from build123d import *

# Parameters (mm, degrees)
F0_W     = 80
F0_H     = 25
F0_R     = 7.5
F1_DEPTH = 5
F2_W     = 80
F2_H     = 25
F2_R     = 7.5
F2_W_2   = 5
F2_H_2   = 5
F3_DEPTH = 5


with BuildPart() as f1:
    # F0 (on Top) → F1 (new body)
    with BuildSketch(Plane.XY):
        with Locations((-49.0031225234, 12.5)):
            Rectangle(F0_W, F0_H)
        with Locations((-21.5031225234, 12.5)):
            Circle(F0_R, mode=Mode.SUBTRACT)
    extrude(amount=F1_DEPTH)

    # F2 (on face) → F3 (join)
    with BuildSketch(Plane(origin=(0, 0, 0), x_dir=(1, 0, 0), z_dir=(0, 0, -1))):
        with Locations((-49.0031225234, -12.5)):
            Rectangle(F2_W, F2_H)
        with Locations((-21.5031225234, -12.5)):
            Circle(F2_R, mode=Mode.SUBTRACT)
        with Locations((-21.5031225234, -12.5)):
            Circle(F2_R)
        with Locations((-21.5031225234, -12.5)):
            Rectangle(F2_W_2, F2_H_2, mode=Mode.SUBTRACT)
    extrude(amount=F3_DEPTH)


solid = f1.part
Geometry check sheet. Reference: the model listing, model coordinates, mm. A direction names the side the tool comes from. Round coordinates to 2 decimals unless told otherwise and drop trailing zeros. Order: outer loops, then holes, each group sorted by start corner. A loop starts at its lowest first (then second) coordinate and runs counter-clockwise, first axis right, second up. Notation, with made-up numbers: M -3.5,-37 L 26.5,-37 A31 cw 26.5,-8 Z; hole C 67.5,-24.5 d9. An arc over 180 degrees is marked long. Write each question's results on one line, items separated by ' | '. Start each with the question number.
1. Cross-section at A-A on y = 12.5. Record the boundary of the cut face in (x, z).
2. Cross-section at C-C on y = 16.5. Record the boundary of the cut face in (x, z), plus the area to 3 significant figures.
3. Draft check along X on faces 1 (the face through (-22, 15, -2)), 2 (the face through (-50, 12, -5)), 3 (the face through (-89.003, 13, 0)). Enter one of: pulls with the +X half, pulls with the -X half, needs draft (parallel to the pull), parting line crosses it, or undercut.
4. Cross-section at B-B on z = 1.75. Record the boundary of the cut face in (x, y), plus the area to 3 significant figures.
5. Material ranges on L1, parallel to Y at x = -23.5, z = 4; L2, parallel to X at y = 14.25, z = 1; L3, parallel to X at y = 16.75, z = 1.75, recorded low to high. Write a range as from..to.
6. Go/stop test with a flat-tipped pin: P1, Ø7.5, axis at x = -19.5, y = 12, coming from the +Z side. Record where the tip stops, or that it passes through.
7. Cross-section at D-D on y = 7.25. Record the boundary of the cut face in (x, z), plus the area to 3 significant figures.
8. Set-up check for faces 4 (the face through (-50, 0, 0)), 5 (the face through (-22, 10, -2)), 6 (the face through (-23.13, 5.18, 2.46)): record each of +Z, -Z, +X, -X, +Y, -Y from which the full face is reachable in a straight line by a thin tool's end or side.
Resolved:
1) outline: M -89,-5 L -24,-5 L -24,0 L -29,0 L -29,5 L -89,5 Z; M -19,-5 L -9,-5 L -9,5 L -14,5 L -14,0 L -19,0 Z
2) outline: M -89,-5 L -9,-5 L -9,5 L -15.16,5 L -15.16,0 L -27.85,0 L -27.85,5 L -89,5 Z | area: 737 mm2
3) face 1: undercut | face 2: needs draft | face 3: pulls with the -X half
4) outline: M -89,0 L -9,0 L -9,25 L -89,25 Z; hole C -21.5,12.5 d15 | area: 1,820 mm2
5) L1: 0..5.27, 19.73..25 | L2: -89..-28.8, -14.21..-9 | L3: -89..-27.68, -15.32..-9
6) P1: z = 0
7) outline: M -89,-5 L -9,-5 L -9,5 L -16.15,5 L -16.15,0 L -26.86,0 L -26.86,5 L -89,5 Z | area: 746 mm2
8) face 4: +Z, -Z, +X, -X, -Y | face 5: +Z, -Z | face 6: +Z
